from build123d import *

# Parameters (mm, degrees)
BOSS_EXTRUDE1_DEPTH = 35
CUT_EXTRUDE1_DEPTH  = 30
CUT_EXTRUDE3_DEPTH  = 5.5
CUT_EXTRUDE4_DEPTH  = 5.5
SKETCH7_R           = 1.5
CUT_EXTRUDE5_DEPTH  = 4
FILLET1_R           = 0.5


with BuildPart() as part:
    # Sketch1 → Boss-Extrude1 (new body)
    with BuildSketch(Plane.XY):
        with BuildLine():
            Line((-7.5, 2.562310746), (7.5, 2.562310746))
            Line((7.5, 2.562310746), (7.5, 11.199242574))
            ThreePointArc((7.5, 11.199242574), (0, 9.562310746), (-7.5, 11.199242574))
            Line((-7.5, 11.199242574), (-7.5, 2.562310746))
        make_face()
    extrude(amount=BOSS_EXTRUDE1_DEPTH)

    # Sketch3 → Cut-Extrude1 (cut)
    with BuildSketch(Plane(origin=(0, 5.562310746, 0), x_dir=(-1, 0, 0), z_dir=(0, -1, 0))):
        with BuildLine():
            Line((-3.5, -3.5), (-3.5, 2.919890279))
            Line((-3.5, 2.919890279), (3.5, 2.919890279))
            Line((3.5, 2.919890279), (3.5, -3.5))
            ThreePointArc((3.5, -3.5), (0, -7), (-3.5, -3.5))
        make_face()
        with BuildLine():
            Line((3.5, -31.5), (3.5, -38.189637839))
            Line((3.5, -38.189637839), (-3.5, -38.189637839))
            Line((-3.5, -38.189637839), (-3.5, -31.5))
            ThreePointArc((-3.5, -31.5), (0, -28), (3.5, -31.5))
        make_face()
    extrude(amount=-CUT_EXTRUDE1_DEPTH, mode=Mode.SUBTRACT)

    # Sketch5 → Cut-Extrude3 (cut)
    with BuildSketch(Plane.XY.offset(7.75)):
        with BuildLine():
            Line((-7.5, 11.199242574), (-7.5, 2.562310746))
            Line((-7.5, 2.562310746), (7.5, 2.562310746))
            Line((7.5, 2.562310746), (7.5, 11.199242574))
            ThreePointArc((7.5, 11.199242574), (0, 5.062310746), (-7.5, 11.199242574))
        make_face()
    extrude(amount=CUT_EXTRUDE3_DEPTH, mode=Mode.SUBTRACT)

    # Sketch6 → Cut-Extrude4 (cut)
    with BuildSketch(Plane.XY.offset(27.25)):
        with BuildLine():
            Line((-7.5, 11.199242574), (-7.5, 2.562310746))
            Line((-7.5, 2.562310746), (7.5, 2.562310746))
            Line((7.5, 2.562310746), (7.5, 11.199242574))
            ThreePointArc((7.5, 11.199242574), (0, 5.062310746), (-7.5, 11.199242574))
        make_face()
    extrude(amount=-CUT_EXTRUDE4_DEPTH, mode=Mode.SUBTRACT)

    # Sketch7 → Cut-Extrude5 (cut, through all)
    with BuildSketch(Plane(origin=(0, 5.562310746, 0), x_dir=(1, 0, 0), z_dir=(0, 1, 0))):
        with Locations((0, -3.5)):
            Circle(SKETCH7_R)
        with Locations((0, -31.5)):
            Circle(SKETCH7_R)
    extrude(amount=-CUT_EXTRUDE5_DEPTH, mode=Mode.SUBTRACT)

    # Fillet1
    fillet1_edges = [part.edges().sort_by_distance(p)[0] for p in [
        (0, 5.062310746, 7.75),
        (0, 5.062310746, 13.25),
        (0, 5.062310746, 21.75),
        (0, 5.062310746, 27.25),
    ]]
    fillet(fillet1_edges, radius=FILLET1_R)


solid = part.part
Design review of the part built by this model. Coordinates are the model's own, in mm. A direction names the side the tool comes from. Coordinates: 2 decimals unless noted, no trailing zeros. Loops run counter-clockwise (first coordinate to the right, second up) from the corner with the lowest first, then second, coordinate; pieces in that order, holes last. Notation, with made-up numbers: (27, 73) -> (49, 73) arc R20 cw to (49, 105) -> close; hole circle Ø10 at (80, 19.25). An arc over 180 degrees is marked (long way). Use a Markdown table: item, result. Add a question column.
Item 1: Wall thickness on L1, parallel to Z at x = 4.25, y = 3.5; L2, parallel to Z at x = 0, y = 4.3; L3, parallel to X at y = 3.95, z = 31.5: over which ranges is each line inside the solid? List them lowest first. Write a range as from..to.
Item 2: We need section B-B, the plane z = 4. Write out the cut boundary in (x, y), and give its area (3 significant figures).
Item 3: We need section A-A, the plane x = 0. Write out the cut boundary in (y, z), and give its area (3 significant figures).
Item 4: We need section C-C, the plane z = 28.5. Write out the cut boundary in (x, y).
Item 5: Clearance check with flat-ended pins moving along their axes: P1, Ø2, axis at x = 1, z = 3, coming from the +Y side; P2, Ø1.5, axis at y = 5, z = 10, coming from the -X side; P3, Ø1, axis at y = 4.5, z = 10, coming from the -X side. State where each tip first meets the part, or that it passes through.
Item 6: Machinability: for faces 5 (the flat face through (0, 4, 7.75)), 6 (the flat face through (1, 5.562, 2)), 7 (the flat face through (1, 5.562, 33)), which of the approach directions +Z, -Z, +X, -X, +Y, -Y give a long, thin tool a straight path to every point of the face, cutting with its end or side? Answer none if there is none.
Item 7: We need section D-D, the plane z = 9.5. Write out the cut boundary in (x, y), and give its area (3 significant figures).
Item 8: The part is to be moulded in two halves that separate along Z. For faces 1 (the flat face through (0, 4, 13.25)), 2 (the cylindrical face through (0, 8, 7)), 3 (the flat face through (3.5, 8, 2)), 4 (the cylindrical face through (0, 8, 28)), say which applies: +Z half, -Z half, draft (parallel to the pull), parting line (faces both ways), or undercut.
Numbers:
| question | item | result |
|---|---|---|
| 1 | L1 | z = 0..7.75, 13.25..21.75, 27.25..35 |
| 1 | L2 | z = 0..2, 5..7.75, 13.25..21.75, 27.25..30, 33..35 |
| 1 | L3 | x = -7.5..-1.5, 1.5..7.5 |
| 2 | outline | (-7.5, 2.56) -> (-1.41, 2.56) -> (-1.41, 5.56) -> (-3.46, 5.56) -> (-3.46, 9.9) arc R18 cw to (-7.5, 11.2) -> close; (1.41, 2.56) -> (7.5, 2.56) -> (7.5, 11.2) arc R18 cw to (3.46, 9.9) -> (3.46, 5.56) -> (1.41, 5.56) -> close |
| 2 | area | 76.1 mm^2 |
| 3 | outline | (2.56, 0) -> (5.56, 0) -> (5.56, 2) -> (2.56, 2) -> close; (2.56, 5) -> (5.56, 5) -> (5.56, 7) -> (9.56, 7) -> (9.56, 28) -> (5.56, 28) -> (5.56, 30) -> (2.56, 30) -> (2.56, 27.25) -> (4.56, 27.25) arc R0.5 cw to (5.06, 26.75) -> (5.06, 22.25) arc R0.5 cw to (4.56, 21.75) -> (2.56, 21.75) -> (2.56, 13.25) -> (4.56, 13.25) arc R0.5 cw to (5.06, 12.75) -> (5.06, 8.25) arc R0.5 cw to (4.56, 7.75) -> (2.56, 7.75) -> close; (2.56, 33) -> (5.56, 33) -> (5.56, 35) -> (2.56, 35) -> close |
| 3 | area | 144 mm^2 |
| 4 | outline | (-7.5, 2.56) -> (7.5, 2.56) -> (7.5, 11.2) arc R18 cw to (1.8, 9.65) -> (1.8, 5.56) -> (-1.8, 5.56) -> (-1.8, 9.65) arc R18 cw to (-7.5, 11.2) -> close |
| 5 | P1 | stops at y = 5.56 |
| 5 | P2 | stops at x = -3.17 |
| 5 | P3 | passes through |
| 6 | face 5 | -Y |
| 6 | face 6 | -Z, +Y |
| 6 | face 7 | +Z, +Y |
| 7 | outline | (-7.5, 11.2) arc R7.65 ccw to (7.5, 11.2) arc R18 cw to start |
| 7 | area | 52.4 mm^2 |
| 8 | face 1 | undercut |
| 8 | face 2 | -Z half |
| 8 | face 3 | draft |
| 8 | face 4 | +Z half |
